CAD build for the part. Positions are in the model's coordinates, mm. Face numbers are marked on the shaded views. A direction names the side the tool comes from. Coordinates: 2 decimals unless noted, no trailing zeros. Write each loop counter-clockwise with the first axis right and the second up, starting at its lowest first coordinate (ties: lowest second). Pieces come first, ordered by that corner, then holes. Notation, with made-up numbers: (-3.75, 61) -> (5.25, 61) arc R31 cw to (5.25, 99) -> close; hole circle Ø4 at (-16.5, -13.5). An arc over 180 degrees is marked (long way). Answer as CSV lines item,"result".
```python
from build123d import *

# Parameters (mm, degrees)
ESQUISSE1_R                         = 60
CYLINDRE_PRINCIPAL_DEPTH            = 6
BOSSAGE_RV_R                        = 45
LOGEMENT_RV_DEPTH                   = 20
ESQUISSE20_R                        = 7.5
BOSS_EXTRU_2_DEPTH                  = 6
TROUS_AV_D                          = 4.5
TROUS_AV_CSINK_D                    = 4.85
TROUS_AV_CSINK_ANGLE                = 90
DIAM_TRE_DU_PER_AGE_4_4_4_4_2_DEPTH = 20
D_AGEMENT_SM_D                      = 6.6
TROU_RECOVERY_D                     = 13.5
TROU_RECOVERY_CSINK_D               = 13.55
TROU_RECOVERY_CSINK_ANGLE           = 90
ESQUISSE40_R                        = 16
ENL_V_MAT_EXTRU_2_DEPTH             = 13
CONG_9_R                            = 2
ESQUISSE15_W                        = 5
ESQUISSE15_H                        = 6
CONG_10_R                           = 2


# Read off the part's stored shape, not the designer's step: Diamètre du perçage Ø4.4 (4.4)2
with BuildPart() as part:
    # Esquisse1 → Cylindre principal (new body)
    with BuildSketch(Plane.XY):
        Circle(ESQUISSE1_R)
    extrude(amount=CYLINDRE_PRINCIPAL_DEPTH)

    # Bossage RV → Logement RV (add)
    with BuildSketch(Plane.XY):
        Circle(BOSSAGE_RV_R)
    extrude(amount=LOGEMENT_RV_DEPTH)

    # Esquisse20 → Boss.-Extru.2 (add)
    with BuildSketch(Plane.XY):
        with Locations((-37.123106012, 37.123106012)):
            Circle(ESQUISSE20_R)
    extrude(amount=BOSS_EXTRU_2_DEPTH)

    # Trous AV (through all)
    with Locations(Plane(origin=(0, 40, 0), x_dir=(-1, 0, 0), z_dir=(0, 0, -1))):
        with Locations((0, 0), (40, -40), (0, -80), (-40, -40)):
            CounterSinkHole(TROUS_AV_D / 2, TROUS_AV_CSINK_D / 2, counter_sink_angle=TROUS_AV_CSINK_ANGLE)

    # Diamètre du perçage Ø4.4 (4.4)2 outline → Diamètre du perçage Ø4.4 (4.4)2 (cut)
    with BuildSketch(Plane.XY):
        with BuildLine():
            ThreePointArc((30.65064108, 4), (28.45064108, 6.2), (26.25064108, 4))
            Line((26.25064108, 4), (26.25064108, -4))
            ThreePointArc((26.25064108, -4), (28.45064108, -6.2), (30.65064108, -4))
            Line((30.65064108, -4), (30.65064108, 4))
        make_face()
    extrude(amount=DIAM_TRE_DU_PER_AGE_4_4_4_4_2_DEPTH, mode=Mode.SUBTRACT)

    # Déagement SM (through all)
    with Locations(Plane.XY.offset(6)):
        with Locations((-37.123106012, 37.123106012)):
            Hole(D_AGEMENT_SM_D / 2)

    # Trou recovery (through all)
    with Locations(Plane(origin=(0, 0, 0), x_dir=(-1, 0, 0), z_dir=(0, 0, -1))):
        with Locations((0, 0)):
            CounterSinkHole(TROU_RECOVERY_D / 2, TROU_RECOVERY_CSINK_D / 2, counter_sink_angle=TROU_RECOVERY_CSINK_ANGLE)

    # Esquisse40 → Enlèv. mat.-Extru.2 (cut)
    with BuildSketch(Plane(origin=(0, 0, 0), x_dir=(-1, 0, 0), z_dir=(0, 0, -1))):
        Circle(ESQUISSE40_R)
    extrude(amount=-ENL_V_MAT_EXTRU_2_DEPTH, mode=Mode.SUBTRACT)

    # Congé9
    cong_9_edges = [part.edges().sort_by_distance(p)[0] for p in [
        (16, 0, 0),
    ]]
    fillet(cong_9_edges, radius=CONG_9_R)

    # Esquisse15 → Trou caméra (revolve, cut)
    with BuildSketch(Plane(origin=(-23.641512829, -24.949340174, 6), x_dir=(0, -1, 0), z_dir=(1, 0, 0))):
        with Locations((2.5, 3)):
            Rectangle(ESQUISSE15_W, ESQUISSE15_H)
    revolve(axis=Axis((-23.641512829, -24.949340174, 12.35), (0, 0, -1)), mode=Mode.SUBTRACT)

    # Congé10
    cong_10_edges = [part.edges().sort_by_distance(p)[0] for p in [
        (16, 0, 13),
    ]]
    fillet(cong_10_edges, radius=CONG_10_R)


solid = part.part
```
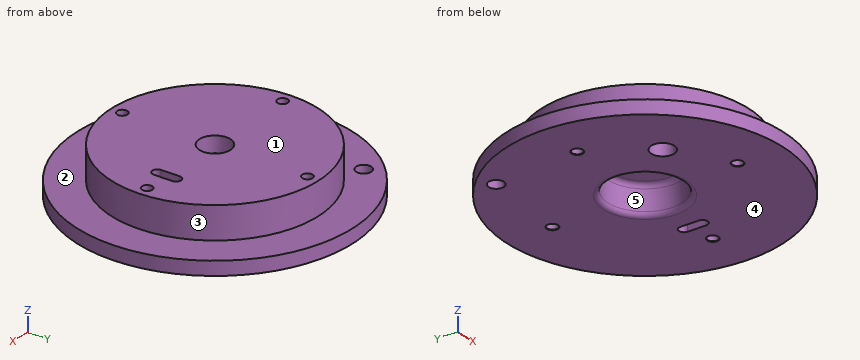
Item 1: Two-plate mould, pull along Y, no slides. Class the marked faces 3, 4 and 5: pulls with the +Y half, pulls with the -Y half, needs draft (parallel to the pull), parting line crosses it, or undercut.
Answer below:
face 3,"parting line crosses it"
face 4,"needs draft"
face 5,"undercut"
Item 2: 3-axis set-ups, long thin cutter, end or side, ignore diameter. For the marked faces 1 and 2: which of +Z, -Z, +X, -X, +Y, -Y reach the whole face in a straight line?
Answer below:
face 1,"+Z, +X, -X, +Y, -Y"
face 2,"+Z"
Item 3: Flat gauge pins, fed straight in: pin 1 (10 mm diameter, centred on y = 40.5, z = 3.5, fed in from +X); pin 2 (2 mm diameter, centred on y = -25, z = 2.5, fed in from +X); pin 3 (5 mm diameter, centred on x = -23.5, y = -23, fed in from -Z). Where does each tip first touch, or does it go through?
Answer below:
pin 1,"stops at x = 48.37"
pin 2,"stops at x = 54.99"
pin 3,"stops at z = 6"
Item 4: Saw through at A-A on x = 0. State how many separate pieces and enclosed holes the cut face has, and give its area (3 significant figures).
Answer below:
separate pieces,"4"
enclosed holes,"0"
area,"1,290 mm2"
Item 5: Wall check: line 1 (Y direction, x = 0, z = 5.75); line 2 (Y direction, x = 0, z = 11.25); line 3 (X direction, y = 5, z = 19). Give the ranges that are in metal, low to high. Write a range as from..to.
Answer below:
line 1,"y = -60..-42.25, -37.75..-16, 16..37.75, 42.25..60"
line 2,"y = -45..-42.25, -37.75..-15.98, 15.98..37.75, 42.25..45"
line 3,"x = -44.72..-4.53, 4.53..26.49, 30.41..44.72"
Item 6: Saw through at C-C on y = -40. Give the cut face in (x, z) (3 decimals).
Answer below:
outline,"(-44.721, 0) -> (-2.425, 0) -> (-2.25, 0.175) -> (-2.25, 20) -> (-20.616, 20) -> (-20.616, 6) -> (-44.721, 6) -> close; (2.25, 0.175) -> (2.425, 0) -> (44.721, 0) -> (44.721, 6) -> (20.616, 6) -> (20.616, 20) -> (2.25, 20) -> close"
Item 7: Saw through at B-B on z = 16. Give the cut face in (x, y).
Answer below:
outline,"circle Ø90 at (0, 0); hole circle Ø4.5 at (-40, 0); hole circle Ø13.5 at (0, 0); hole circle Ø4.5 at (0, -40); hole circle Ø4.5 at (0, 40); hole (26.25, -4) arc R2.2 ccw to (30.65, -4) -> (30.65, 4) arc R2.2 ccw to (26.25, 4) -> close; hole circle Ø4.5 at (40, 0)"
